from build123d import *

# Parameters (mm, degrees)
F0_R     = 3.175
F0_R_2   = 1.5875
F1_DEPTH = 25.4


with BuildPart() as f1:
    # F0 (on Front) → F1 (new body)
    with BuildSketch(Plane.XZ):
        with BuildLine():
            ThreePointArc((15.0877196672, 58.5627598555), (15.6769444522, 61.0001924791), (15.875, 63.5))
            ThreePointArc((15.875, 63.5), (15.8430821396, 64.5061676396), (15.7474569047, 65.5082893304))
            Line((15.7474569047, 65.5082893304), (15.0877196672, 58.5627598555))
        make_face()
        with BuildLine():
            Line((15.0877196672, 58.5627598555), (15.7474569047, 65.5082893304))
            ThreePointArc((15.7474569047, 65.5082893304), (0, 79.375), (-15.7474569047, 65.5082893304))
            Line((-15.7474569047, 65.5082893304), (-15.0877196672, 58.5627598555))
            ThreePointArc((-15.0877196672, 58.5627598555), (0, 47.625), (15.0877196672, 58.5627598555))
        make_face()
        with Locations((0, 63.5)):
            Circle(F0_R, mode=Mode.SUBTRACT)
        with BuildLine():
            ThreePointArc((-15.7474569047, 65.5082893304), (0, 79.375), (15.7474569047, 65.5082893304))
            Line((15.7474569047, 65.5082893304), (9.525, 114.3))
            ThreePointArc((9.525, 114.3), (0, 104.775), (-9.525, 114.3))
            Line((-9.525, 114.3), (-15.7474569047, 65.5082893304))
        make_face()
        with Locations((-3.3911804203, 99.949)):
            Circle(F0_R_2, mode=Mode.SUBTRACT)
        with BuildLine():
            Line((11.1919966494, 17.549675393), (15.0877196672, 58.5627598555))
            ThreePointArc((15.0877196672, 58.5627598555), (0, 47.625), (-15.0877196672, 58.5627598555))
            Line((-15.0877196672, 58.5627598555), (-9.525, 0))
            ThreePointArc((-9.525, 0), (0, 9.525), (9.525, 0))
            ThreePointArc((9.525, 0), (6.9712901065, -6.4905114784), (0.6794904459, -9.5007324841))
            Line((0.6794904459, -9.5007324841), (44.45, -7.9375))
            ThreePointArc((44.45, -7.9375), (36.5125, 0), (44.45, 7.9375))
            Line((44.45, 7.9375), (18.8228170321, 8.8527565346))
            ThreePointArc((18.8228170321, 8.8527565346), (13.130598856, 11.5544736108), (11.1919966494, 17.549675393))
        make_face()
        with BuildLine():
            Line((-15.0877196672, 58.5627598555), (-15.7474569047, 65.5082893304))
            ThreePointArc((-15.7474569047, 65.5082893304), (-15.8038641944, 61.9988332792), (-15.0877196672, 58.5627598555))
        make_face()
        with BuildLine():
            ThreePointArc((-9.525, 114.3), (0, 104.775), (9.525, 114.3))
            ThreePointArc((9.525, 114.3), (0, 123.825), (-9.525, 114.3))
        make_face()
        with Locations((0, 114.3)):
            Circle(F0_R, mode=Mode.SUBTRACT)
        with BuildLine():
            ThreePointArc((9.525, 0), (0, 9.525), (-9.525, 0))
            ThreePointArc((-9.525, 0), (-6.7351920908, -6.7351920908), (0, -9.525))
            Line((0, -9.525), (0.6794904459, -9.5007324841))
            ThreePointArc((0.6794904459, -9.5007324841), (6.9712901065, -6.4905114784), (9.525, 0))
        make_face()
        Circle(F0_R, mode=Mode.SUBTRACT)
        with BuildLine():
            Line((0.6794904459, -9.5007324841), (0, -9.525))
            ThreePointArc((0, -9.525), (0.3399618281, -9.5189311877), (0.6794904459, -9.5007324841))
        make_face()
        with BuildLine():
            ThreePointArc((52.3875, 0), (50.0626600757, 5.6126600757), (44.45, 7.9375))
            ThreePointArc((44.45, 7.9375), (36.5125, 0), (44.45, -7.9375))
            ThreePointArc((44.45, -7.9375), (50.0626600757, -5.6126600757), (52.3875, 0))
        make_face()
        with Locations((44.45, 0)):
            Circle(F0_R, mode=Mode.SUBTRACT)
    extrude(amount=F1_DEPTH)


solid = f1.part
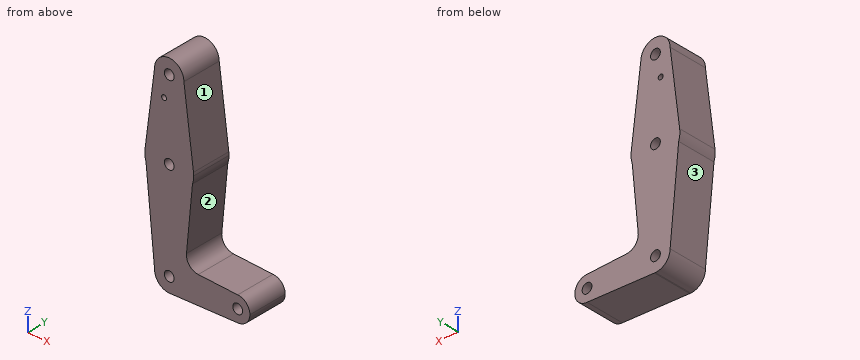
Read the model definition and answer for the solid it produces. Units are mm, in the model's axes. Face numbers are marked on the shaded views. Give positions to 0.01 mm unless a question says otherwise; leave off trailing zeros. Write each loop counter-clockwise with the first axis right and the second up, starting at its lowest first coordinate (ties: lowest second). Pieces come first, ordered by that corner, then holes. Notation, with made-up numbers: (41, 56) - (94, 56) arc R13 ccw to (94, 79) - close; hole circle Ø3 at (-32, 56). An arc over 180 degrees is marked (long way). Use CSV: the item, a comma, the result in double quotes. Start each with the question number.
(1) Determine the mould class of the marked faces 1, 2 and 3 for opening direction Z: +Z half, -Z half, draft (parallel to the pull), parting line (faces both ways), or undercut.
(2) Find section C-C (x = 27). Give the vertices of the cut face in (y, z).
(3) Consider line 1 along Z through (x, y) = (0, -8) (3 decimals); line 2 along X through (y, z) = (-2.75, 1); line 3 along X through (y, z) = (-3, 2). Determine where each line is inside the solid, lowest interval first.
(4) Find section A-A (y = -9.75). Count the separate pieces of the cut face and the enclosed holes in it, plus the area to 3 significant figures.
(5) Given P1, Ø8, axis at x = 28.5, y = -2.5, coming from the +Z side; P2, Ø3, axis at x = 18.5, y = -16, coming from the -Z side; P3, Ø3, axis at y = -11, z = 71, coming from the -X side, each flat-ended and moving along its own axis, determine where each tip first touches the part or whether it passes through.
(6) Find section B-B (z = 54). Give the vertices of the cut face in (x, y).
Findings below:
1,face 1,"+Z half"
1,face 2,"undercut"
1,face 3,"-Z half"
2,outline,"(-25.4, -8.56) - (0, -8.56) - (0, 8.56) - (-25.4, 8.56) - close"
3,line 1,"-9.525 to -3.175, 3.175 to 60.325, 66.675 to 111.125, 117.475 to 123.825"
3,line 2,"-9.62 to -3.01, 3.01 to 41.44, 47.46 to 52.32"
3,line 3,"-9.71 to -2.47, 2.47 to 41.98, 46.92 to 52.13"
4,separate pieces,"1"
4,enclosed holes,"5"
4,area,"3,770 mm2"
5,P1,"z = 8.65"
5,P2,"z = -8.92"
5,P3,"x = -15.24"
6,outline,"(-14.65, -25.4) - (14.65, -25.4) - (14.65, 0) - (-14.65, 0) - close"
